CAD build for the part. Positions are in the model's coordinates, mm. Coordinates: 2 decimals unless noted, no trailing zeros. Write each loop counter-clockwise with the first axis right and the second up, starting at its lowest first coordinate (ties: lowest second). Pieces come first, ordered by that corner, then holes.
```python
from build123d import *

# Parameters (mm, degrees)
SKIZZE1_W                       = 60
SKIZZE1_H                       = 50
AUFSATZ_LINEAR_AUSTRAGEN1_DEPTH = 20
SKIZZE2_R                       = 2.5
SCHNITT_LINEAR_AUSTRAGEN1_DEPTH = 12


with BuildPart() as part:
    # Skizze1 → Aufsatz-Linear austragen1 (new body)
    with BuildSketch(Plane.XY):
        Rectangle(SKIZZE1_W, SKIZZE1_H)
    extrude(amount=AUFSATZ_LINEAR_AUSTRAGEN1_DEPTH)

    # Skizze2 → Schnitt-Linear austragen1 (cut)
    with BuildSketch(Plane.XY.offset(20)):
        with Locations((10, 10)):
            Circle(SKIZZE2_R)
    extrude(amount=-SCHNITT_LINEAR_AUSTRAGEN1_DEPTH, mode=Mode.SUBTRACT)


solid = part.part
```
Item 1: Wall check: line 1 along Y through (x, z) = (10, 16.5); line 2 along Y through (x, z) = (9, 10.75). Give the ranges that are in metal, low to high.
Item 2: Two-plate mould, pull along Y, no slides. Class faces 1 (the cylindrical face through (9.46, 7.56, 14.08)), 2 (the flat face through (10, 10, 8)), 3 (the flat face through (0, 25, 10)), 4 (the flat face through (0, 0, 0)): +Y half, -Y half, draft (parallel to the pull), parting line (faces both ways), or undercut.
Item 3: Flat gauge pins, fed straight in: pin 1 Ø1.5 at (x, y) = (22.5, 0.5) entering from -Z; pin 2 Ø4 at (x, y) = (10, 10) entering from +Z. Where does each tip first touch, or does it go through?
Item 4: Saw through at B-B, the plane x = 10. Write the cut outline in (y, z), and give its area (3 significant figures).
Item 5: Saw through at A-A, the plane y = 10. Write the cut outline in (x, z), and give its area (3 significant figures).
Working result:
1. line 1: y = -25 to 7.5, 12.5 to 25
1. line 2: y = -25 to 7.71, 12.29 to 25
2. face 1: undercut
2. face 2: undercut
2. face 3: +Y half
2. face 4: draft
3. pin 1: stops at z = 0
3. pin 2: stops at z = 8
4. outline: (-25, 0) - (25, 0) - (25, 20) - (12.5, 20) - (12.5, 8) - (7.5, 8) - (7.5, 20) - (-25, 20) - close
4. area: 940 mm2
5. outline: (-30, 0) - (30, 0) - (30, 20) - (12.5, 20) - (12.5, 8) - (7.5, 8) - (7.5, 20) - (-30, 20) - close
5. area: 1,140 mm2
